```python
from build123d import *

# Parameters (mm, degrees)
SKETCH1_R             = 60
SKETCH1_R_2           = 58.8
BOSS_EXTRUDE1_DEPTH   = 20
SKETCH1_R_3           = 10
BOSS_EXTRUDE1_2_DEPTH = 20
BOSS_EXTRUDE4_DEPTH   = 20
CIRPATTERN1_COUNT     = 8
SKETCH2_R             = 16
SKETCH2_R_2           = 15
BOSS_EXTRUDE2_DEPTH   = 20
BOSS_EXTRUDE3_DEPTH   = 20


with BuildPart() as part:
    # Sketch1 → Boss-Extrude1 (new body)
    with BuildSketch(Plane(origin=(0, 0, 0), x_dir=(1, 0, 0), z_dir=(0, 1, 0))):
        with Locations(Location((0, 0, 0), (0, 0, 270))):
            Circle(SKETCH1_R)
        with Locations(Location((0, 0, 0), (0, 0, 270))):
            Circle(SKETCH1_R_2, mode=Mode.SUBTRACT)
    extrude(amount=BOSS_EXTRUDE1_DEPTH)



with BuildPart() as body_2:
    # Sketch1 → Boss-Extrude1 2 (new body)
    with BuildSketch(Plane(origin=(0, 0, 0), x_dir=(1, 0, 0), z_dir=(0, 1, 0))):
        with Locations(Location((0, 0, 0), (0, 0, 270))):
            Circle(SKETCH1_R_3)
        with BuildLine():
            ThreePointArc((2.603003073, -3.2), (0, 4.125), (-2.603003073, -3.2))
            Line((-2.603003073, -3.2), (2.603003073, -3.2))
        make_face(mode=Mode.SUBTRACT)
    extrude(amount=BOSS_EXTRUDE1_2_DEPTH)


with BuildPart() as part_1:
    add(part.part)

    add(body_2.part)  # Boss-Extrude4 merges body 2
    # Sketch4 → Boss-Extrude4 (add)
    with BuildSketch(Plane(origin=(0, 0, 0), x_dir=(1, 0, 0), z_dir=(0, 1, 0))):
        with BuildLine():
            Line((-9.632475442, -0.71058124), (-10, 0))
            ThreePointArc((-10, 0), (-26.841730813, -33.640288469), (0, -60))
            Line((0, -60), (0.117199585, -59.208631402))
            ThreePointArc((0.117199585, -59.208631402), (-26.052615674, -33.508769279), (-9.632475442, -0.71058124))
        make_face()
    boss_extrude4 = extrude(amount=BOSS_EXTRUDE4_DEPTH)

    # CirPattern1: Boss-Extrude4 ×8 about axis
    cirpattern1_axis = Axis((0, 0, 0), (0, 1, 0))
    for i in range(1, CIRPATTERN1_COUNT):
        add(boss_extrude4.rotate(cirpattern1_axis, i * 360 / CIRPATTERN1_COUNT))

    # Sketch2 → Boss-Extrude2 (add)
    with BuildSketch(Plane(origin=(0, 0, 0), x_dir=(1, 0, 0), z_dir=(0, 1, 0))):
        Circle(SKETCH2_R)
        Circle(SKETCH2_R_2, mode=Mode.SUBTRACT)
    extrude(amount=BOSS_EXTRUDE2_DEPTH)

    # Sketch3 → Boss-Extrude3 (add)
    with BuildSketch(Plane(origin=(0, 0, 0), x_dir=(1, 0, 0), z_dir=(0, 1, 0))):
        with BuildLine():
            Line((0, -68), (0, -60))
            ThreePointArc((0, -60), (-6.139084092, -59.685104059), (-12.213729096, -58.74372155))
            ThreePointArc((-12.213729096, -58.74372155), (-5.063374474, -61.994967767), (0, -68))
        make_face()
        with BuildLine():
            ThreePointArc((42.426406871, -42.426406871), (37.862753824, -46.544729808), (32.901673193, -50.174494528))
            ThreePointArc((32.901673193, -50.174494527), (40.256715681, -47.417408534), (48.083261121, -48.08326112))
            Line((48.083261121, -48.08326112), (42.426406871, -42.426406871))
        make_face()
        with BuildLine():
            Line((-48.083261121, -48.083261121), (-42.426406872, -42.426406871))
            ThreePointArc((-42.426406871, -42.426406871), (-46.544729808, -37.862753824), (-50.174494528, -32.901673193))
            ThreePointArc((-50.174494528, -32.901673193), (-47.417408535, -40.256715682), (-48.083261121, -48.083261121))
        make_face()
        with BuildLine():
            ThreePointArc((60, 0), (59.685104059, -6.139084092), (58.74372155, -12.213729095))
            ThreePointArc((58.74372155, -12.213729095), (61.994967767, -5.063374474), (68, 1e-09))
            Line((68, 1e-09), (60, 1e-09))
        make_face()
        with BuildLine():
            Line((-68.000000001, 0), (-60.000000001, 0))
            ThreePointArc((-60, 0), (-59.685104059, 6.139084092), (-58.74372155, 12.213729096))
            ThreePointArc((-58.743721551, 12.213729096), (-61.994967768, 5.063374474), (-68.000000001, 0))
        make_face()
        with BuildLine():
            ThreePointArc((42.42640687, 42.426406872), (46.544729807, 37.862753825), (50.174494527, 32.901673194))
            ThreePointArc((50.174494527, 32.901673194), (47.417408534, 40.256715682), (48.08326112, 48.083261122))
            Line((48.08326112, 48.083261122), (42.42640687, 42.426406872))
        make_face()
        with BuildLine():
            Line((-48.083261122, 48.083261121), (-42.426406872, 42.426406871))
            ThreePointArc((-42.426406872, 42.426406871), (-37.862753824, 46.544729807), (-32.901673194, 50.174494527))
            ThreePointArc((-32.901673194, 50.174494528), (-40.256715682, 47.417408534), (-48.083261122, 48.083261121))
        make_face()
        with BuildLine():
            ThreePointArc((-1e-09, 60), (6.139084091, 59.685104059), (12.213729095, 58.74372155))
            ThreePointArc((12.213729095, 58.743721551), (5.063374473, 61.994967768), (-1e-09, 68.000000001))
            Line((-1e-09, 68.000000001), (-1e-09, 60.000000001))
        make_face()
    extrude(amount=BOSS_EXTRUDE3_DEPTH)


solid = part_1.part
```
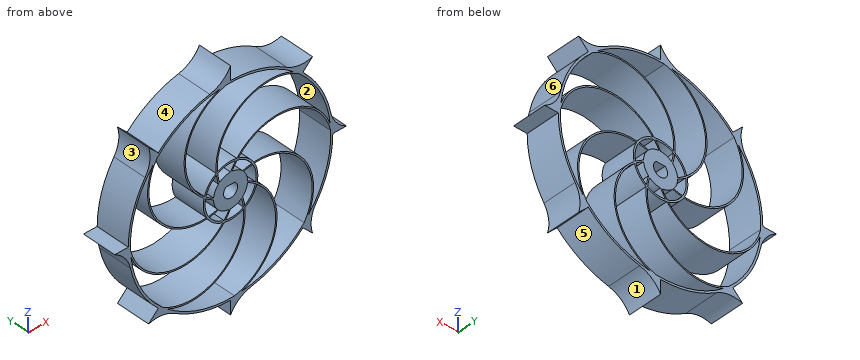
Can you work these out from the model? Positions are in its coordinate system, mm. Face numbers are marked on the shaded views. A direction names the side the tool comes from. Coordinates: 2 decimals unless noted, no trailing zeros. Write each loop counter-clockwise with the first axis right and the second up, starting at its lowest first coordinate (ties: lowest second). Pieces come first, ordered by that corner, then holes. Notation, with made-up numbers: (73, 58) - (84, 58) arc R15 ccw to (84, 76) - close; hole circle Ø4 at (63.5, -34). An arc over 180 degrees is marked (long way). Return JSON: item names as keys, results as strings.
Q1. If we section it at B-B (y = 4): Count the separate pieces of the cut face and the enclosed holes in it, then the cut area to 3 significant figures.
Computed values:
{"separate pieces": "1", "enclosed holes": "17", "area": "1,510 mm2"}
Q2. Please list where these lines run through material, in increasing order: L1, parallel to Z at x = -35.5, y = 15.5; L2, parallel to Z at x = -31.5, y = 1.75. Write a range as from..to.
Computed values:
{"L1": "z = -48.76..-46.87, -46.33..-45.47, -26.47..-25.65, -2.51..-1.51, 46.87..48.37", "L2": "z = -51.07..-49.65, -47.67..-46.84, -27.12..-26.32, -4.97..-4.07, 49.65..51.07"}
Q3. If we section it at A-A (z = 54): Please give me the cut outline in (x, y), then the cut area to 3 significant figures.
Computed values:
{"outline": "(-26.15, 0) - (-23.27, 0) - (-23.27, 20) - (-26.15, 20) - close; (-14.43, 0) - (-13.06, 0) - (-13.06, 20) - (-14.43, 20) - close; (23.27, 0) - (26.15, 0) - (26.15, 20) - (23.27, 20) - close", "area": "143 mm2"}
Q4. Thinking about a two-plate mould opening in X: for the marked faces 1, 2 and 3, which applies, +X half, -X half, draft (parallel to the pull), parting line (faces both ways), or undercut?
Computed values:
{"face 1": "+X half", "face 2": "undercut", "face 3": "-X half"}
Q5. I'm going to push flat-ended pins straight in: pin 1 Ø2.5 at (y, z) = (9.5, 63.5) entering from +X; pin 2 Ø4 at (y, z) = (6.5, -64) entering from -X; pin 3 Ø2 at (x, y) = (15, 10.5) entering from +Z; pin 4 Ø13 at (x, z) = (0, 0) entering from +Y. Where does each tip first touch, or does it pass through?
Computed values:
{"pin 1": "stops at x = 0", "pin 2": "stops at x = 0", "pin 3": "stops at z = 58.34", "pin 4": "stops at y = 20"}
Q6. On a 3-axis mill with a long thin cutter (end or side, diameter ignored), from which of +Z, -Z, +X, -X, +Y, -Y can I reach the whole of each face in a straight line? I mean the marked faces 4, 5 and 6. Say none if no direction works.
Computed values:
{"face 4": "+Z, +Y, -Y", "face 5": "-Z, +Y, -Y", "face 6": "+X, +Y, -Y"}
